Autodesk Inventor part; units mm, degrees
ref_plane "YZ Plane" through (0, 0, 0) normal (1, 0, 0) x (0, 1, 0)
ref_plane "XZ Plane" through (0, 0, 0) normal (0, 1, 0) x (-1, 0, 0)
ref_plane "XY Plane" through (0, 0, 0) normal (0, 0, 1) x (1, 0, 0)
sketch "Sketch1" plane through (0, 0, 0) normal (0, 1, 0) x (-1, 0, 0)
  point P0 (0, 0)
sketch "Sketch2" plane through (0, 0, 0) normal (0, 1, 0) x (-1, 0, 0)
  line L0 (23.5, 27) -> (-23.5, 27)
  line L1 (-23.5, 27) -> (-23.5, -27)
  line L2 (-23.5, -27) -> (23.5, -27)
  line L3 (23.5, -27) -> (23.5, 27)
  dimension "d4" = 47
  dimension "d5" = 54
extrude "Extrusion1" add sketch "Sketch2" along normal blind 2
sketch "Sketch3" plane through (0, 2, 0) normal (0, 1, 0) x (1, 0, 0)
  point P0 (0, 0)
sketch "Sketch4" plane through (0, 2, 0) normal (0, 1, 0) x (1, 0, 0)
  circle A0 centre (19.5, 22.5) radius 1.5
  circle A1 centre (19.5, -22.5) radius 1.5
  circle A2 centre (-19.5, -22.5) radius 1.5
  circle A3 centre (-19.5, 22.5) radius 1.5
  circle A4 centre (-19.5, 22.5) radius 2.25
  circle A5 centre (19.5, 22.5) radius 2.25
  circle A6 centre (19.5, -22.5) radius 2.25
  circle A7 centre (-19.5, -22.5) radius 2.25
  dimension "d24" = 3
  dimension "d27" = 3
  dimension "d30" = 3
  dimension "d33" = 3
  dimension "d34" = 4.5
  dimension "d35" = 4.5
  dimension "d36" = 4.5
  dimension "d37" = 4.5
extrude "Extrusion2" add sketch "Sketch4" along normal blind 3
sketch "Sketch5" plane through (0, 2, 0) normal (0, 1, 0) x (1, 0, 0)
  circle A0 centre (-17.5, -17.5) radius 2
  circle A1 centre (-17.5, 17.5) radius 2
  circle A2 centre (17.5, 17.5) radius 2
  circle A3 centre (17.5, -17.5) radius 2
  dimension "d42" = 4
  dimension "d43" = 4
  dimension "d44" = 4
  dimension "d45" = 4
extrude "Extrusion3" cut sketch "Sketch5" against normal through all
properties part number "Box1_Buttom"
Input: part model. Units: mm. Frame: model coordinates. A direction names the side the tool comes from. Round coordinates to 2 decimals unless told otherwise and drop trailing zeros. Write each loop counter-clockwise with the first axis right and the second up, starting at its lowest first coordinate (ties: lowest second). Pieces come first, ordered by that corner, then holes.
1) Reachability of faces 4 (the flat face through (20, 2, 23)), 5 (the flat face through (0, 0, 0)) from +Z, -Z, +X, -X, +Y, -Y: full face, straight path, thin tool, end or side. Return the list, or none.
2) Cut plane B-B (z = -17.5). Return the cut outline in (x, y), then the cut area to 3 significant figures.
3) Draft query along X for faces 1 (the flat face through (-23.5, 1, 0)), 2 (the cylindrical face through (-17.76, 1.014, -19.483)), 3 (the flat face through (0, 1, 27)). Return one class per face: pulls with the +X half, pulls with the -X half, needs draft (parallel to the pull), parting line crosses it, or undercut.
4) Contact query for flat-ended pins moving along their axis: P1, Ø4, axis at x = 0, z = -11, coming from the -Y side; P2, Ø14, axis at x = -9, z = 8.5, coming from the +Y side. Output: stop coordinate, or through.
5) Cut plane D-D (x = -1). Return the cut outline in (y, z), then the cut area to 3 significant figures.
6) Cut plane C-C (x = 16.5). Return the cut outline in (y, z).
7) Ray query, L1, parallel to X at y = 1.6, z = 17.5; L2, parallel to X at y = 3.9, z = -22.5; L3, parallel to Z at x = 17.5, y = 0.5. Return the intervals inside material, ascending.
8) Cut plane A-A (y = 3.6). Return the cut outline in (x, z), then the cut area to 3 significant figures.
Geometry says:
1. face 4: +Y
1. face 5: +Z, -Z, +X, -X, -Y
2. outline: (-23.5, 0) - (-19.5, 0) - (-19.5, 2) - (-23.5, 2) - close; (-15.5, 0) - (15.5, 0) - (15.5, 2) - (-15.5, 2) - close; (19.5, 0) - (23.5, 0) - (23.5, 2) - (19.5, 2) - close
2. area: 78.0 mm2
3. face 1: pulls with the -X half
3. face 2: undercut
3. face 3: needs draft
4. P1: stops at y = 0
4. P2: stops at y = 2
5. outline: (0, -27) - (2, -27) - (2, 27) - (0, 27) - close
5. area: 108 mm2
6. outline: (0, -27) - (2, -27) - (2, -19.23) - (0, -19.23) - close; (0, -15.77) - (2, -15.77) - (2, 15.77) - (0, 15.77) - close; (0, 19.23) - (2, 19.23) - (2, 27) - (0, 27) - close
7. L1: x = -23.5 to -19.5, -15.5 to 15.5, 19.5 to 23.5
7. L2: x = -21.75 to -21, -18 to -17.25, 17.25 to 18, 21 to 21.75
7. L3: z = -27 to -19.5, -15.5 to 15.5, 19.5 to 27
8. outline: circle Ø4.5 at (-19.5, -22.5); circle Ø4.5 at (-19.5, 22.5); circle Ø4.5 at (19.5, -22.5); circle Ø4.5 at (19.5, 22.5); hole circle Ø3 at (-19.5, -22.5); hole circle Ø3 at (-19.5, 22.5); hole circle Ø3 at (19.5, -22.5); hole circle Ø3 at (19.5, 22.5)
8. area: 35.3 mm2
